from build123d import *

# Parameters (mm, degrees)
F0_W      = 60
F0_H      = 33
F1_DEPTH  = 160
F2_W      = 30
F2_H      = 123
F3_DEPTH  = 60.001
F4_W      = 21
F4_H      = 123
F5_DEPTH  = 33.001
F7_W      = 57
F7_H      = 27
F8_DEPTH  = 3
F9_W      = 21
F9_H      = 37
F10_DEPTH = 30


with BuildPart() as f1:
    # F0 (on Top) → F1 (new body)
    with BuildSketch(Plane.XY):
        Rectangle(F0_W, F0_H)
    extrude(amount=F1_DEPTH)

    # F2 (on face) → F3 (cut, through all)
    with BuildSketch(Plane(origin=(-30, 0, 0), x_dir=(0, -1, 0), z_dir=(-1, 0, 0))):
        with Locations((1.5, 61.5)):
            Rectangle(F2_W, F2_H)
    extrude(amount=-F3_DEPTH, mode=Mode.SUBTRACT)

    # F4 (on face) → F5 (cut, through all)
    with BuildSketch(Plane(origin=(0, 16.5, 0), x_dir=(-1, 0, 0), z_dir=(0, 1, 0))):
        with Locations((0, -61.5)):
            Rectangle(F4_W, F4_H)
        with Locations((0, 61.5)):
            Rectangle(F4_W, F4_H)
    extrude(amount=-F5_DEPTH, mode=Mode.SUBTRACT)

    # F7 (on offset) → F8 (cut)
    with BuildSketch(Plane.XY.offset(123)):
        Rectangle(F7_W, F7_H)
    extrude(amount=F8_DEPTH, mode=Mode.SUBTRACT)

    # F9 (on face) → F10 (join)
    with BuildSketch(Plane(origin=(0, 16.5, 0), x_dir=(-1, 0, 0), z_dir=(0, 1, 0))):
        Polygon((30, 0), (30, 160), (10.5, 160), (10.5, 123), (10.5, 0), align=None)
        with Locations((0, 141.5)):
            Rectangle(F9_W, F9_H)
        Polygon((-10.5, 123), (-10.5, 160), (-30, 160), (-30, 0), (-10.5, 0), align=None)
    extrude(amount=F10_DEPTH)


solid = f1.part
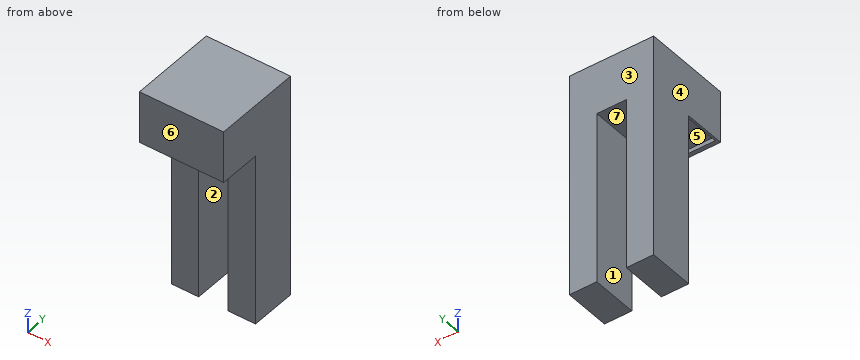
CAD build for the part. Positions are in the model's coordinates, mm. Face numbers are marked on the shaded views. A direction names the side the tool comes from. Give positions to 0.01 mm unless a question says otherwise; leave off trailing zeros. Order: outer loops, then holes, each group sorted by start corner. A loop starts at its lowest first (then second) coordinate and runs counter-clockwise, first axis right, second up. Notation, with made-up numbers: (-35, 54) -> (18, 54) arc R18 ccw to (18, 79) -> close; hole circle Ø7 at (37.5, 63). An arc over 180 degrees is marked (long way). Return JSON: item names as keys, results as strings.
Q1. Flat gauge pins, fed straight in: pin 1 (6.5 mm diameter, centred on x = 0.5, y = 30.5, fed in from -Z); pin 2 (1.5 mm diameter, centred on x = 18.5, z = 71, fed in from -Y). Where does each tip first touch, or does it go through?
Working result:
{"pin 1": "z = 123", "pin 2": "y = 13.5"}
Q2. Drill centre lines: line 1 (X direction, y = 23, z = 72); line 2 (Z direction, x = -23, y = 1); line 3 (Y direction, x = -17.5, z = 12). Where is each one in solid material? Low to high.
Working result:
{"line 1": "-30 to -10.5, 10.5 to 30", "line 2": "126 to 160", "line 3": "13.5 to 46.5"}
Q3. Saw through at A-A (z = 78.5). Write the cut outline in (x, y).
Working result:
{"outline": "(-30, 13.5) -> (-10.5, 13.5) -> (-10.5, 46.5) -> (-30, 46.5) -> close; (10.5, 13.5) -> (30, 13.5) -> (30, 46.5) -> (10.5, 46.5) -> close"}
Q4. Which spindle directions (+Z, -Z, +X, -X, +Y, -Y) get a long thin tool onto all of the face, cutting with end or side? Do the marked faces 5, 6 and 7. Say none if no direction does.
Working result:
{"face 5": "-Z", "face 6": "+Z, -Z, +X, -X, -Y", "face 7": "-Z, +Y, -Y"}
Q5. Saw through at B-B (x = 14). Write the cut outline in (y, z), then the cut area to 3 significant figures.
Working result:
{"outline": "(-16.5, 123) -> (-13.5, 123) -> (-13.5, 126) -> (13.5, 126) -> (13.5, 0) -> (46.5, 0) -> (46.5, 160) -> (-16.5, 160) -> close", "area": "6,310 mm²"}
Q6. Mould opens along X. For the marked faces 1, 2, 3 and 4 say: pulls with the +X half, pulls with the -X half, needs draft (parallel to the pull), parting line crosses it, or undercut.
Working result:
{"face 1": "undercut", "face 2": "undercut", "face 3": "needs draft", "face 4": "pulls with the -X half"}
Q7. Saw through at C-C (y = -10). Write the cut outline in (x, z).
Working result:
{"outline": "(-30, 123) -> (-28.5, 123) -> (-28.5, 126) -> (28.5, 126) -> (28.5, 123) -> (30, 123) -> (30, 160) -> (-30, 160) -> close"}
